Can you work these out from the model? Positions are in its coordinate system, mm. A direction names the side the tool comes from. Coordinates: 2 decimals unless noted, no trailing zeros. Order: outer loops, then holes, each group sorted by start corner. A loop starts at its lowest first (then second) coordinate and runs counter-clockwise, first axis right, second up. Notation, with made-up numbers: (42, 81) - (84, 81) arc R16 cw to (84, 103) - close; hole circle Ø9 at (62, 82). An arc over 180 degrees is marked (long way). Return JSON: item names as keys, results as strings. Group by question number.
1) Imagine slicing it at B-B (x = 10.5). Write out the boundary of the cut face in (y, z), and give its area (3 significant figures).
2) If we mould it in two halves opening along Y, with no side actions, what happens to faces 1 (the face through (-66.844, -39.223, 1.014)), 2 (the face through (75.464, 44.293, 0.986)), 3 (the face through (-75.464, -44.293, 0.986))? For each: pulls with the +Y half, pulls with the -Y half, needs draft (parallel to the pull), parting line crosses it, or undercut.
3) Imagine slicing it at C-C (y = -56.5). Write out the boundary of the cut face in (x, z), and give its area (3 significant figures).
4) For pin 1 Ø1 at (y, z) = (-18, 0.5) entering from +X, with a flat end and sliding along its axis, tell me the tip position at first contact or that it passes through.
5) Which directions (+Z, -Z, +X, -X, +Y, -Y) give clear straight access to the entire face, cutting with the end or side of a thin tool? Please do faces 4 (the face through (67.39, -38.28, 1.01)), 5 (the face through (76.09, -43.21, 0.99)).
6) Imagine slicing it at A-A (z = 0.95). Write out the boundary of the cut face in (x, y), and give its area (3 significant figures).
7) If I drill on line 1 along Y through (x, z) = (-8.5, 0.1); line 2 along X through (y, z) = (-58, 1.35); line 3 along X through (y, z) = (-35, 0.3), over which ranges is the centre line in solid material (lowest first)?
Autodesk Inventor part; units mm, degrees
ref_plane "YZ Plane" through (0, 0, 0) normal (1, 0, 0) x (0, 1, 0)
ref_plane "XZ Plane" through (0, 0, 0) normal (0, 1, 0) x (-1, 0, 0)
ref_plane "XY Plane" through (0, 0, 0) normal (0, 0, 1) x (1, 0, 0)
sketch "Sketch1" plane through (0, 0, 0) normal (0, 0, 1) x (1, 0, 0)
  line L0 (50.5181, -87.5) -> (-50.5181, -87.5)
  line L1 (-50.5181, -87.5) -> (-101.0363, 0)
  line L2 (-101.0363, 0) -> (-50.5181, 87.5)
  line L3 (-50.5181, 87.5) -> (50.5181, 87.5)
  line L4 (50.5181, 87.5) -> (101.0363, 0)
  line L5 (101.0363, 0) -> (50.5181, -87.5)
  point P0 (0, 0)
  point P1 (0, 0)
  dimension "d0" = 175
extrude "Extrusion1" add sketch "Sketch1" along normal blind 2
sketch "Sketch7" plane through (0, 0, 2) normal (0, 0, 1) x (1, 0, 0)
  line L0 (-50.5181, -87.5) -> (50.5181, -87.5)
  line L1 (50.5181, -87.5) -> (101.0363, 0)
  line L2 (101.0363, 0) -> (50.5181, 87.5)
  line L3 (50.5181, 87.5) -> (-50.5181, 87.5)
  line L4 (-50.5181, 87.5) -> (-101.0363, 0)
  line L5 (-101.0363, 0) -> (-50.5181, -87.5)
  line L6 (-44.7446, 77.5) -> (44.7446, 77.5)
  line L7 (44.7446, 77.5) -> (89.4893, 0)
  line L8 (89.4893, 0) -> (44.7446, -77.5)
  line L9 (44.7446, -77.5) -> (-44.7446, -77.5)
  line L10 (-44.7446, -77.5) -> (-89.4893, 0)
  line L11 (-89.4893, 0) -> (-44.7446, 77.5)
  dimension "d26" = 10
extrude "Extrusion6" cut sketch "Sketch7" against normal blind 7 contours L6 L7 L8 L9 L10 L11
fillet "Fillet2" radius 10 6 edges at (-89.4893, 0, 1) (-44.7446, -77.5, 1) (44.7446, -77.5, 1) (89.4893, 0, 1) (44.7446, 77.5, 1) (-44.7446, 77.5, 1)
fillet "Fillet3" radius 10 6 edges at (-50.5181, 87.5, 1) (50.5181, 87.5, 1) (101.0363, 0, 1) (50.5181, -87.5, 1) (-50.5181, -87.5, 1) (-101.0363, 0, 1)
properties part number "Cover v1"
Calculated:
{
 "1": {"outline": "(-87.5, 0) - (-77.5, 0) - (-77.5, 2) - (-87.5, 2) - close; (77.5, 0) - (87.5, 0) - (87.5, 2) - (77.5, 2) - close", "area": "40.0 mm2"},
 "2": {"face 1": "undercut", "face 2": "pulls with the +Y half", "face 3": "pulls with the -Y half"},
 "3": {"outline": "(-68.42, 0) - (-56.87, 0) - (-56.87, 2) - (-68.42, 2) - close; (56.87, 0) - (68.42, 0) - (68.42, 2) - (56.87, 2) - close", "area": "46.2 mm2"},
 "4": {"pin 1": "x = 90.93"},
 "5": {"face 4": "+Z, -Z", "face 5": "+Z, -Z, +X, -Y"},
 "6": {"outline": "(-98.15, -5) - (-53.4, -82.5) arc R10 ccw to (-44.74, -87.5) - (44.74, -87.5) arc R10 ccw to (53.4, -82.5) - (98.15, -5) arc R10 ccw to (98.15, 5) - (53.4, 82.5) arc R10 ccw to (44.74, 87.5) - (-44.74, 87.5) arc R10 ccw to (-53.4, 82.5) - (-98.15, 5) arc R10 ccw to start; hole (-86.6, -5) - (-47.63, -72.5) arc R10 ccw to (-38.97, -77.5) - (38.97, -77.5) arc R10 ccw to (47.63, -72.5) - (86.6, -5) arc R10 ccw to (86.6, 5) - (47.63, 72.5) arc R10 ccw to (38.97, 77.5) - (-38.97, 77.5) arc R10 ccw to (-47.63, 72.5) - (-86.6, 5) arc R10 ccw to start", "area": "5,720 mm2"},
 "7": {"line 1": "-87.5 to -77.5, 77.5 to 87.5", "line 2": "-67.55 to -56, 56 to 67.55", "line 3": "-80.83 to -69.28, 69.28 to 80.83"}
}
